from build123d import *

# Parameters (mm, degrees)
SKETCH3_R           = 2
SKETCH3_R_2         = 1.5
SKETCH3_R_3         = 4
BOSS_EXTRUDE1_DEPTH = 2
SKETCH6_W           = 19.838520206
SKETCH6_H           = 2.488043404
CUT_EXTRUDE1_DEPTH  = 50


with BuildPart() as part:
    # Sketch3 → Boss-Extrude1 (new body)
    with BuildSketch(Plane(origin=(0, 0, 0), x_dir=(1, 0, 0), z_dir=(0, 1, 0))):
        with BuildLine():
            Line((17, 13), (-30, 13))
            Line((-30, 13), (-30, -13))
            Line((-30, -13), (17, -13))
            ThreePointArc((17, -13), (30, 0), (17, 13))
        make_face()
        with Locations(Location((-24.346479472, -6.5, 0), (0, 0, 270))):
            Circle(SKETCH3_R, mode=Mode.SUBTRACT)
        with Locations(Location((-9.346479472, -6.5, 0), (0, 0, 270))):
            Circle(SKETCH3_R, mode=Mode.SUBTRACT)
        with Locations(Location((-9.346479472, 6.5, 0), (0, 0, 270))):
            Circle(SKETCH3_R, mode=Mode.SUBTRACT)
        with Locations(Location((-24.346479472, 6.5, 0), (0, 0, 270))):
            Circle(SKETCH3_R, mode=Mode.SUBTRACT)
        with Locations(Location((17, -8.5, 0), (0, 0, 270))):
            Circle(SKETCH3_R_2, mode=Mode.SUBTRACT)
        with Locations(Location((17, 8.5, 0), (0, 0, 270))):
            Circle(SKETCH3_R_2, mode=Mode.SUBTRACT)
        with Locations(Location((17, 0, 0), (0, 0, 270))):
            Circle(SKETCH3_R_3, mode=Mode.SUBTRACT)
    extrude(amount=BOSS_EXTRUDE1_DEPTH)

    # Sketch6 → Cut-Extrude1 (cut)
    with BuildSketch(Plane(origin=(0, 2, 0), x_dir=(1, 0, 0), z_dir=(0, 1, 0))):
        with Locations((-2, 0)):
            Rectangle(SKETCH6_W, SKETCH6_H)
    extrude(amount=-CUT_EXTRUDE1_DEPTH, mode=Mode.SUBTRACT)


solid = part.part
CAD build for the part. Positions are in the model's coordinates, mm. A direction names the side the tool comes from. Round coordinates to 2 decimals unless told otherwise and drop trailing zeros. Order: outer loops, then holes, each group sorted by start corner. A loop starts at its lowest first (then second) coordinate and runs counter-clockwise, first axis right, second up. Notation, with made-up numbers: (10.5, -19.5) - (23.5, -19.5) arc R27 cw to (23.5, -0.5) - close; hole circle Ø8 at (-18.5, 82.5). An arc over 180 degrees is marked (long way). Return JSON: item names as keys, results as strings.
(1) Pull direction X, two halves, no side cores. Call faces 1 (the face through (0, 0, -3)), 2 (the face through (-30, 1, 0)), 3 (the face through (30, 1, 0)), 4 (the face through (-2, 1, 1.244)): +X half, -X half, draft (parallel to the pull), parting line (faces both ways), or undercut.
Answer key:
{"face 1": "draft", "face 2": "-X half", "face 3": "+X half", "face 4": "undercut"}
(2) Tool access for faces 5 (the face through (-2, 1, -1.244)), 6 (the face through (-7, 1, 13)): list every direction of +Z, -Z, +X, -X, +Y, -Y with a clear straight run to the whole face (end or side of a thin tool).
Answer key:
{"face 5": "+Y, -Y", "face 6": "+Z, +X, -X, +Y, -Y"}
(3) Cut at A-A (z = 0). Give the cut face in (x, y), then the cut area to 3 significant figures.
Answer key:
{"outline": "(-30, 0) - (-11.92, 0) - (-11.92, 2) - (-30, 2) - close; (7.92, 0) - (13, 0) - (13, 2) - (7.92, 2) - close; (21, 0) - (30, 0) - (30, 2) - (21, 2) - close", "area": "64.3 mm^2"}
(4) Pin check, flat tip, straight feed: pin 1 Ø2.5 at (x, z) = (17, -8.5) entering from -Y. Stop position of the tip, or through.
Answer key:
{"pin 1": "passes through"}
(5) Wall check: probe 1 along X at (y, z) = (1.75, 0); probe 2 along Z at (x, y) = (1.5, 1.95); probe 3 along X at (y, z) = (1.6, -8.25). Give the ranges that are in metal, low to high. Write a range as from..to.
Answer key:
{"probe 1": "x = -30..-11.92, 7.92..13, 21..30", "probe 2": "z = -13..-1.24, 1.24..13", "probe 3": "x = -30..-25.31, -23.38..-10.31, -8.38..15.52, 18.48..27.05"}
(6) Cut at B-B (x = -4). Give the cut face in (y, z).
Answer key:
{"outline": "(0, -13) - (2, -13) - (2, -1.24) - (0, -1.24) - close; (0, 1.24) - (2, 1.24) - (2, 13) - (0, 13) - close"}
(7) Cut at D-D (z = -6.25). Give the cut face in (x, y), then the cut area to 3 significant figures.
Answer key:
{"outline": "(-30, 0) - (-26.33, 0) - (-26.33, 2) - (-30, 2) - close; (-22.36, 0) - (-11.33, 0) - (-11.33, 2) - (-22.36, 2) - close; (-7.36, 0) - (28.4, 0) - (28.4, 2) - (-7.36, 2) - close", "area": "101 mm^2"}
(8) Cut at C-C (y = 0.7). State how many separate pieces and enclosed holes the cut face has, then the cut area to 3 significant figures.
Answer key:
{"separate pieces": "1", "enclosed holes": "8", "area": "1,320 mm^2"}
